Design review of the part built by this model. Coordinates are the model's own, in mm. A direction names the side the tool comes from. Coordinates: 2 decimals unless noted, no trailing zeros. Loops run counter-clockwise (first coordinate to the right, second up) from the corner with the lowest first, then second, coordinate; pieces in that order, holes last. Notation, with made-up numbers: (78, 0.25) -> (126, 0.25) arc R12 ccw to (126, 22.25) -> close; hole circle Ø9 at (-32, 8.25). An arc over 180 degrees is marked (long way). Use a Markdown table: item, result. Add a question column.
Q1. Take a section at D-D on z = 10.25. Write out the cut boundary in (x, y), plus the area to 3 significant figures.
Q2. Take a section at C-C on y = 1. Write out the cut boundary in (x, z), plus the area to 3 significant figures.
Q3. Draft analysis for pull direction Z (two halves, no side actions). For faces 4 (the face through (0, 9, 0)), 5 (the face through (11, 6, 8)), 6 (the face through (0, 11, 6)), state which applies: pulls with the +Z half, pulls with the -Z half, needs draft (parallel to the pull), parting line crosses it, or undercut.
Q4. Take a section at B-B on y = 4.25. Write out the cut boundary in (x, z), plus the area to 3 significant figures.
Q5. For probe 1 along X at (y, z) = (9.55, 6); probe 2 along Z at (x, y) = (-6.5, 5.75); probe 3 along X at (y, z) = (3.5, 10.5), list the stretches that pass through material, from the lowest coordinate up.
Q6. For faces 1 (the face through (-11, 6, 8)), 2 (the face through (7.37, 4.39, 10.03)), 3 (the face through (14.972, 6, 3)), list the 3-axis set-ups (+Z, -Z, +X, -X, +Y, -Y) from which the entire face can be reached by the end or side of a thin tool; tool diameter is ignored.
Q7. Clearance check with flat-ended pins moving along their axes: pin 1 Ø6 at (x, z) = (-7.5, 5.5) entering from -Y; pin 2 Ø2 at (x, z) = (-10.03, 6) entering from +Y; pin 3 Ø2 at (x, z) = (-11.5, 10) entering from -Y; pin 4 Ø3 at (x, z) = (-3.5, 6) entering from -Y. State where each tip first meets the part, or that it passes through.
Q8. Take a section at A-A on z = 6. Write out the cut boundary in (x, y).
Autodesk Inventor part; units mm, degrees
ref_plane "YZ Plane" through (0, 0, 0) normal (1, 0, 0) x (0, 1, 0)
ref_plane "XZ Plane" through (0, 0, 0) normal (0, 1, 0) x (-1, 0, 0)
ref_plane "XY Plane" through (0, 0, 0) normal (0, 0, 1) x (1, 0, 0)
sketch "Szkic1" plane through (0, 0, 0) normal (0, 0, 1) x (1, 0, 0)
  line L0 (-15.0276, 11) -> (14.9724, 11)
  line L1 (14.9724, 11) -> (14.9724, 0)
  line L2 (14.9724, 0) -> (-15.0276, 0)
  line L3 (-15.0276, 0) -> (-15.0276, 11)
  point P0 (0, 0)
  dimension "d0" = 30
  dimension "d1" = 11
extrude "Wyciągnięcie proste1" add sketch "Szkic1" along normal blind 12
sketch "Szkic2" plane through (0, 0, 12) normal (0, 0, 1) x (1, 0, 0)
  line L0 (14.9724, 11) -> (-15.0276, 11)
  line L1 (-0.0276, 11) -> (0, 0)
  line L2 (-15.0276, 11) -> (-15.0276, 0)
  line L3 (-15.0276, 0) -> (14.9724, 0)
  line L4 (-15.0276, 8.66) -> (14.9724, 8.66)
  line L5 (14.9724, 0) -> (14.9724, 11)
  line L6 (-15.0276, 0) -> (-0.0276, 8.66)
  line L7 (-0.0276, 8.66) -> (14.9724, 0)
  line L8 (14.9724, 0) -> (-15.0276, 0)
  dimension "d4" = 8.66
extrude "Wyciągnięcie proste2" cut sketch "Szkic2" against normal blind 12 contours L7 L3 L1 | L1 L3 L6
sketch "Szkic3" plane through (-15.0276, 11, 0) normal (-1, 0, 0) x (0, 0, 1)
  line L0 (12, -2.34) -> (0, -2.34)
  line L1 (0, 0) -> (12, 0)
  line L2 (6, 0) -> (6, -11)
  line L3 (0, -11) -> (12, -11)
  line L4 (8, -2.34) -> (4, -2.34)
  line L5 (4, -2.34) -> (4, -11)
  line L6 (4, -11) -> (8, -11)
  line L7 (8, -11) -> (8, -2.34)
  point P0 (4, -2.34)
  dimension "d7" = 4
extrude "Wyciągnięcie proste3" cut sketch "Szkic3" against normal blind 30
sketch "Szkic4" plane through (-15.0276, 11, 0) normal (0, 1, 0) x (1, 0, 0)
  line L0 (0, 0) -> (0, -12)
  line L1 (0, -6) -> (30, -6)
  line L2 (30, 0) -> (30, -12)
  line L3 (30, -12) -> (0, -12)
  line L4 (25, -12) -> (25, 0)
  line L5 (30, 0) -> (15, 0)
  line L6 (15, -12) -> (15, -8)
  line L7 (15, 0) -> (15, -12)
  line L8 (5, -12) -> (5, 0)
  point P0 (15.0276, 0)
  point P1 (5, -6)
  point P2 (25, -6)
  dimension "d10" = 5
hole "Otwór1" at (-10.0276, 11, 6) at (9.9724, 11, 6) direction (0, -1, 0) diameter 2.459 depth 8.8 tip angle 118
properties part number "szczęka" material "Stal nierdzewna 440C"
Answer list:
| question | item | result |
|---|---|---|
| 1 | outline | (-15.03, 0) -> (-0.03, 8.66) -> (14.97, 0) -> (14.97, 11) -> (-15.03, 11) -> close |
| 1 | area | 200 mm² |
| 2 | outline | (-15.03, 0) -> (-13.3, 0) -> (-13.3, 4) -> (-15.03, 4) -> close; (-15.03, 8) -> (-13.3, 8) -> (-13.3, 12) -> (-15.03, 12) -> close; (13.24, 0) -> (14.97, 0) -> (14.97, 4) -> (13.24, 4) -> close; (13.24, 8) -> (14.97, 8) -> (14.97, 12) -> (13.24, 12) -> close |
| 2 | area | 27.7 mm² |
| 3 | face 4 | pulls with the -Z half |
| 3 | face 5 | undercut |
| 3 | face 6 | needs draft |
| 4 | outline | (-15.03, 0) -> (-7.67, 0) -> (-7.67, 4) -> (-15.03, 4) -> close; (-15.03, 8) -> (-7.67, 8) -> (-7.67, 12) -> (-15.03, 12) -> close; (7.61, 0) -> (14.97, 0) -> (14.97, 4) -> (7.61, 4) -> close; (7.61, 8) -> (14.97, 8) -> (14.97, 12) -> (7.61, 12) -> close |
| 4 | area | 118 mm² |
| 5 | probe 1 | -15.03 to -11.26, -8.8 to 8.74, 11.2 to 14.97 |
| 5 | probe 2 | 0 to 4, 8 to 12 |
| 5 | probe 3 | -15.03 to -8.97, 8.91 to 14.97 |
| 6 | face 1 | +X, -X, -Y |
| 6 | face 2 | +Z, -Z, -Y |
| 6 | face 3 | +Z, -Z, +X, +Y, -Y |
| 7 | pin 1 | y = 2.85 |
| 7 | pin 2 | through |
| 7 | pin 3 | y = 1.46 |
| 7 | pin 4 | y = 8.66 |
| 8 | outline | (-15.03, 8.66) -> (-11.26, 8.66) -> (-11.26, 11) -> (-15.03, 11) -> close; (-8.8, 8.66) -> (8.74, 8.66) -> (8.74, 11) -> (-8.8, 11) -> close; (11.2, 8.66) -> (14.97, 8.66) -> (14.97, 11) -> (11.2, 11) -> close |
